The listing builds one solid part. Answer for the finished solid, in the listing's coordinates (mm). Give positions to 0.01 mm unless a question says otherwise; leave off trailing zeros. Write each loop counter-clockwise with the first axis right and the second up, starting at its lowest first coordinate (ties: lowest second). Pieces come first, ordered by that corner, then holes. Notation, with made-up numbers: M 47,-7.5 L 80,-7.5 A23 ccw 80,23.5 Z; hole C 6,-9.5 d7. An arc over 180 degrees is marked long. Return JSON: item names as keys, results as strings.
Autodesk Inventor part; units mm, degrees
ref_plane "YZ Plane" through (0, 0, 0) normal (1, 0, 0) x (0, 1, 0)
ref_plane "XZ Plane" through (0, 0, 0) normal (0, 1, 0) x (-1, 0, 0)
ref_plane "XY Plane" through (0, 0, 0) normal (0, 0, 1) x (1, 0, 0)
sketch "Skizze1" plane through (0, 0, 0) normal (0, 1, 0) x (-1, 0, 0)
  line L0 (31.1765, -16.3235) -> (11.1765, -16.3235)
  line L1 (11.1765, -16.3235) -> (11.1765, -36.3235)
  line L2 (11.1765, -36.3235) -> (31.1765, -36.3235)
  line L3 (31.1765, -36.3235) -> (31.1765, -16.3235)
  point P0 (0, 0)
  dimension "d0" = 20
  dimension "d1" = 20
extrude "Extrusion1" add sketch "Skizze1" along normal blind 300
sketch "Skizze2" plane through (0, 0, 0) normal (0, -1, 0) x (1, 0, 0)
  line L0 (-11.1765, -16.3235) -> (-11.1765, -36.3235)
  line L1 (-31.1765, -16.3235) -> (-11.1765, -16.3235)
  circle A0 centre (-21.1765, -26.3235) radius 2.5676
  point P0 (0, 0)
  dimension "d5" = 10
  dimension "d6" = 10
extrude "Extrusion2" add sketch "Skizze2" along normal blind 20
sketch "Skizze3" plane through (0, 300, 0) normal (0, 1, 0) x (1, 0, 0)
  line L0 (-11.1765, 16.3235) -> (-11.1765, 36.3235)
  line L1 (-11.1765, 23.8235) -> (-16.1765, 23.8235)
  line L2 (-16.1765, 23.8235) -> (-16.1765, 28.8235)
  line L3 (-16.1765, 28.8235) -> (-11.1765, 28.8235)
  line L4 (-11.1765, 28.8235) -> (-11.1765, 23.8235)
  line L5 (-11.1765, 36.3235) -> (-31.1765, 36.3235)
  line L6 (-23.6765, 36.3235) -> (-18.6765, 36.3235)
  line L7 (-18.6765, 36.3235) -> (-18.6765, 31.3235)
  line L8 (-18.6765, 31.3235) -> (-23.6765, 31.3235)
  line L9 (-23.6765, 31.3235) -> (-23.6765, 36.3235)
  line L10 (-31.1765, 23.8235) -> (-26.1765, 23.8235)
  line L11 (-26.1765, 23.8235) -> (-26.1765, 28.8235)
  line L12 (-26.1765, 28.8235) -> (-31.1765, 28.8235)
  line L13 (-31.1765, 28.8235) -> (-31.1765, 23.8235)
  line L14 (-31.1765, 16.3235) -> (-11.1765, 16.3235)
  line L15 (-23.6765, 16.3235) -> (-18.6765, 16.3235)
  line L16 (-18.6765, 16.3235) -> (-18.6765, 21.3235)
  line L17 (-18.6765, 21.3235) -> (-23.6765, 21.3235)
  line L18 (-23.6765, 21.3235) -> (-23.6765, 16.3235)
  line L19 (-31.1765, 36.3235) -> (-31.1765, 16.3235)
  point P0 (0, 0)
  dimension "d9" = 5
  dimension "d10" = 7.5
  dimension "d11" = 7.5
  dimension "d12" = 5
  dimension "d13" = 7.5
  dimension "d14" = 5
  dimension "d15" = 5
  dimension "d16" = 7.5
  dimension "d17" = 5
  dimension "d18" = 5
  dimension "d19" = 5
  dimension "d20" = 5
extrude "Extrusion3" cut sketch "Skizze3" against normal blind 300 contours L1 L2 L3 L0 | L14 L18 L17 L16 | L7 L8 L9 L5 | L13 L12 L11 L10
properties material "Aluminium 6061"
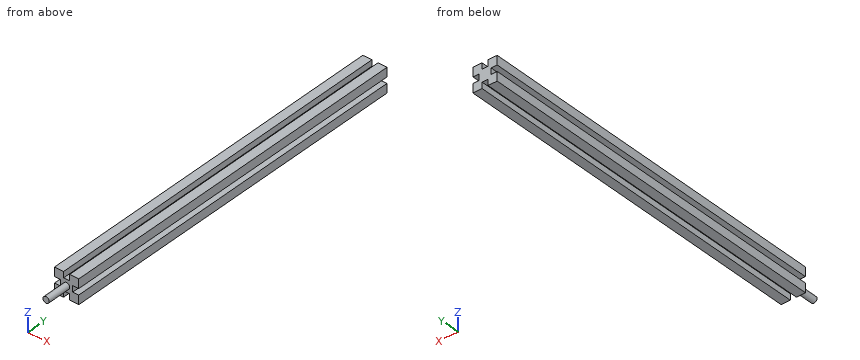
Item 1: A cutting plane is placed at A-A, the plane y = 186. Write down the section's boundary in (x, z), plus the area to 3 significant figures.
Geometry results:
{"outline": "M -31.18,-36.32 L -23.68,-36.32 L -23.68,-31.32 L -18.68,-31.32 L -18.68,-36.32 L -11.18,-36.32 L -11.18,-28.82 L -16.18,-28.82 L -16.18,-23.82 L -11.18,-23.82 L -11.18,-16.32 L -18.68,-16.32 L -18.68,-21.32 L -23.68,-21.32 L -23.68,-16.32 L -31.18,-16.32 L -31.18,-23.82 L -26.18,-23.82 L -26.18,-28.82 L -31.18,-28.82 Z", "area": "300 mm2"}
Item 2: Find the intervals of material crossed by line 1 (X direction, y = 106, z = -34.5); line 2 (Z direction, x = -26.25, y = 280); line 3 (Y direction, x = -28, z = -32), in increasing order.
Geometry results:
{"line 1": "x = -31.18 to -23.68, -18.68 to -11.18", "line 2": "z = -36.32 to -28.82, -23.82 to -16.32", "line 3": "y = 0 to 300"}
Item 3: Given pin 1 Ø5 at (y, z) = (210, -25.5) entering from -X; pin 2 Ø1.5 at (x, y) = (-20.5, 210.5) entering from -Z; pin 3 Ø1.5 at (y, z) = (216.5, -26) entering from +X, each flat-ended and moving along its own axis, determine where each tip first touches the part or whether it passes through.
Geometry results:
{"pin 1": "stops at x = -31.18", "pin 2": "stops at z = -31.32", "pin 3": "stops at x = -16.18"}
